CAD build for the part. Positions are in the model's coordinates, mm. A direction names the side the tool comes from. Coordinates: 2 decimals unless noted, no trailing zeros. Order: outer loops, then holes, each group sorted by start corner. A loop starts at its lowest first (then second) coordinate and runs counter-clockwise, first axis right, second up. Notation, with made-up numbers: (13, 71) - (50, 71) arc R16 ccw to (50, 80) - close; hole circle Ø11 at (33, -19). An arc over 180 degrees is marked (long way). Return JSON: item names as keys, results as strings.
from build123d import *

# Parameters (mm, degrees)
F1_DEPTH     = 10.25
F3_DEPTH     = 2.25
F4_R         = 1
F5_T         = 1.9
F5_T3_DEPTH  = 4.8
F5_T5_DEPTH  = 28.8
F5_T8_ANGLE  = 90.000000001
F5_T10_ANGLE = 90.000000001


# Not quite as in the source:
# - a shell that OpenCascade refuses in one call is made with other operations: the cavity is built on its own and cut out


with BuildPart() as f1:
    # F0 (on Top) → F1 (new body)
    with BuildSketch(Plane.XY):
        with BuildLine():
            ThreePointArc((24, 11), (21.6568542495, 16.6568542495), (16, 19))
            Line((16, 19), (-16, 19))
            ThreePointArc((-16, 19), (-21.6568542495, 16.6568542495), (-24, 11))
            Line((-24, 11), (-24, -11))
            ThreePointArc((-24, -11), (-21.6568542495, -16.6568542495), (-16, -19))
            Line((-16, -19), (16, -19))
            ThreePointArc((16, -19), (21.6568542495, -16.6568542495), (24, -11))
            Line((24, -11), (24, 11))
        make_face()
    extrude(amount=F1_DEPTH)

    # F2 (on face) → F3 (join)
    with BuildSketch(Plane.XY.offset(10.25)):
        with BuildLine():
            Line((8, 21.85), (-16, 21.85))
            ThreePointArc((-16, 21.85), (-21.6568542495, 19.5068542495), (-24, 13.85))
            Line((-24, 13.85), (-24, -13.85))
            ThreePointArc((-24, -13.85), (-21.6568542495, -19.5068542495), (-16, -21.85))
            Line((-16, -21.85), (8, -21.85))
            ThreePointArc((8, -21.85), (8.7071067812, -21.5571067812), (9, -20.85))
            Line((9, -20.85), (9, 20.85))
            ThreePointArc((9, 20.85), (8.7071067812, 21.5571067812), (8, 21.85))
        make_face()
    extrude(amount=-F3_DEPTH)

    # F4
    f4_edges = [f1.edges().sort_by_distance(p)[0] for p in [
        (9, -19, 9.125),
        (9, 19, 9.125),
    ]]
    fillet(f4_edges, radius=F4_R)

    # F5: shell of thickness 1.9, made by hand


with BuildPart() as f5_core1:
    # F5_t2: copy of F1
    add(f1.part)

    # the walls: a layer under each face that stays
    f5_faces = [f5_core1.faces().sort_by_distance(p)[0] for p in [
        (0, 0, 10.25),
        (0, 19, 5.125),
        (9.2928932188, 19.2928932188, 9.125),
        (21.6568542495, 16.6568542495, 5.125),
        (9, 20.425, 9.125),
        (24, 0, 5.125),
        (21.6568542495, -16.6568542495, 5.125),
        (-4, 21.85, 9.125),
        (0, -19, 5.125),
        (-21.6568542495, 19.5068542495, 9.125),
        (9.2928932188, -19.2928932188, 9.125),
        (-24, 0, 5.125),
        (9, -20.425, 9.125),
        (-21.6568542495, -19.5068542495, 9.125),
        (-4, -21.85, 9.125),
        (-18.3333333333, 20.0416666667, 8),
        (-21.6568542495, 16.6568542495, 4),
        (-18.3333333333, -20.0416666667, 8),
        (-21.6568542495, -16.6568542495, 4),
    ]]
    thicken(f5_faces, amount=-F5_T, mode=Mode.SUBTRACT)

    # F5_s4 → F5_t3 (cut)
    with BuildSketch(Plane.YZ.offset(7.1)):
        Polygon((19.019, 7.981), (17.1, 8), (17.1, 9.9), (19, 9.9), align=None)
        Polygon((-19.019, 7.981), (-17.1, 8), (-17.1, 9.9), (-19, 9.9), align=None)
    extrude(amount=F5_T3_DEPTH, mode=Mode.SUBTRACT)

    # F5_s6 → F5_t5 (cut)
    with BuildSketch(Plane.YZ.offset(-17.9)):
        Polygon((19.019, 7.981), (17.1, 8), (17.1, 9.9), (19, 9.9), align=None)
        Polygon((-19.019, 7.981), (-17.1, 8), (-17.1, 9.9), (-19, 9.9), align=None)
    extrude(amount=F5_T5_DEPTH, mode=Mode.SUBTRACT)

    # F5_s7 → F5_t8 (revolve, cut)
    with BuildSketch(Plane.XZ.offset(-11)):
        Polygon((-24.019, 7.981), (-24, 9.9), (-22.1, 9.9), (-22.1, 8), align=None)
    revolve(axis=Axis((-16, 11, 8), (0, 0, -1)), revolution_arc=F5_T8_ANGLE, mode=Mode.SUBTRACT)

    # F5_s9 → F5_t10 (revolve, cut)
    with BuildSketch(Plane.YZ.offset(-16)):
        Polygon((-19.019, 7.981), (-19, 9.9), (-17.1, 9.9), (-17.1, 8), align=None)
    revolve(axis=Axis((-16, -11, 8), (0, 0, -1)), revolution_arc=F5_T10_ANGLE, mode=Mode.SUBTRACT)


with BuildPart() as f1_1:
    add(f1.part)

    # what is left inside the walls is the cavity
    f5_cavity = [f5_core1.part.solids().sort_by_distance(p)[0] for p in [
        (0, -5.7, 8.331),
    ]]
    add(f5_cavity, mode=Mode.SUBTRACT)


solid = f1_1.part
Item 1: Mould opens along X. For faces 4 (the cylindrical face through (20.266, -15.361, 4.117)), 5 (the flat face through (-24, 0, 5)), 6 (the flat face through (-4, 21.85, 9)), 7 (the cylindrical face through (20.361, 15.266, 4.117)) say: released by +X, released by -X, zero draft, split by the parting line, or undercut.
Findings below:
{"face 4": "undercut", "face 5": "released by -X", "face 6": "zero draft", "face 7": "undercut"}
Item 2: Band-saw the part on B-B, the plane z = 9. List the corners of the cut face in (x, y).
Findings below:
{"outline": "(-24, -13.85) arc R8 ccw to (-16, -21.85) - (8, -21.85) arc R1 ccw to (9, -20.85) - (9, -20) arc R1 cw to (10, -19) - (16, -19) arc R8 ccw to (24, -11) - (24, 11) arc R8 ccw to (16, 19) - (10, 19) arc R1 cw to (9, 20) - (9, 20.85) arc R1 ccw to (8, 21.85) - (-16, 21.85) arc R8 ccw to (-24, 13.85) - close"}
Item 3: Wall check: L1, parallel to Y at x = -6, z = 3.5; L2, parallel to X at y = -10, z = 1.75; L3, parallel to Z at x = 1.5, y = -6.5. Give the ranges that are in metal, low to high. Write a range as [from, to].
Findings below:
{"L1": "y = [-19, -17.1], [17.1, 19]", "L2": "x = [-24, -22.1], [22.1, 24]", "L3": "z = [8.35, 10.25]"}
Item 4: Band-saw the part on C-C, the plane z = 2.5. List the corners of the cut face in (x, y).
Findings below:
{"outline": "(-24, -11) arc R8 ccw to (-16, -19) - (16, -19) arc R8 ccw to (24, -11) - (24, 11) arc R8 ccw to (16, 19) - (-16, 19) arc R8 ccw to (-24, 11) - close; hole (-22.1, -11) arc R6.1 ccw to (-16, -17.1) - (16, -17.1) arc R6.1 ccw to (22.1, -11) - (22.1, 11) arc R6.1 ccw to (16, 17.1) - (-16, 17.1) arc R6.1 ccw to (-22.1, 11) - close"}
Item 5: Drop flat-ended pins along their axis: P1, Ø1, axis at y = -16.5, z = 3.5, coming from the +X side (3 decimals); P2, Ø1, axis at y = 12, z = 3, coming from the -X side; P3, Ø0.9, axis at y = 20.5, z = 9.5, coming from the +X side. Give the stop position or say it passes through.
Findings below:
{"P1": "stops at x = 22.245", "P2": "stops at x = -23.98", "P3": "stops at x = 9"}
Item 6: Which spindle directions (+Z, -Z, +X, -X, +Y, -Y) get a long thin tool onto all of the face, cutting with end or side? Do faces 1 (the cylindrical face through (-21.719, -16.594, 3.944)), 2 (the flat face through (0, -17.1, 4)), 3 (the cylindrical face through (-21.594, 16.719, 3.944)). Say none if no direction does.
Findings below:
{"face 1": "-Z, -X, -Y", "face 2": "-Z", "face 3": "-Z, -X, +Y"}
Item 7: Band-saw the part on D-D, the plane y = -2.5. List the corners of the cut face in (x, z), then the cut area to 3 significant figures.
Findings below:
{"outline": "(-24, 0) - (-22.1, 0) - (-22.1, 8.35) - (22.1, 8.35) - (22.1, 0) - (24, 0) - (24, 10.25) - (-24, 10.25) - close", "area": "123 mm²"}
Item 8: Band-saw the part on A-A, the plane x = 11.5. List the corners of the cut face in (y, z).
Findings below:
{"outline": "(-19, 0) - (-17.1, 0) - (-17.1, 8.35) - (17.1, 8.35) - (17.1, 0) - (19, 0) - (19, 10.25) - (-19, 10.25) - close"}
